```python
from build123d import *

# Parameters (mm, degrees)
SKETCH1_R           = 1.3335
SKETCH1_R_2         = 1.5875
BOSS_EXTRUDE1_DEPTH = 1.651
CHAMFER1_SIZE       = 2.54
SKETCH5_R           = 4.191
CUT_EXTRUDE5_DEPTH  = 23.382376376


with BuildPart() as part:
    # Sketch1 → Boss-Extrude1 (new body)
    with BuildSketch(Plane(origin=(0, 0, 0), x_dir=(1, 0, 0), z_dir=(0, 1, 0))):
        with BuildLine():
            Line((-5.567119422, 8.9535), (5.567119422, 8.9535))
            ThreePointArc((5.567119422, 8.9535), (6.35, 6.5405), (7.132880578, 8.9535))
            Line((7.132880578, 8.9535), (20.447, 8.9535))
            Line((20.447, 8.9535), (20.447, -8.9535))
            Line((20.447, -8.9535), (7.132880578, -8.9535))
            ThreePointArc((7.132880578, -8.9535), (6.35, -6.5405), (5.567119422, -8.9535))
            Line((5.567119422, -8.9535), (-5.567119422, -8.9535))
            ThreePointArc((-5.567119422, -8.9535), (-6.35, -6.5405), (-7.132880578, -8.9535))
            Line((-7.132880578, -8.9535), (-20.447, -8.9535))
            Line((-20.447, -8.9535), (-20.447, 8.9535))
            Line((-20.447, 8.9535), (-7.132880578, 8.9535))
            ThreePointArc((-7.132880578, 8.9535), (-6.35, 6.5405), (-5.567119422, 8.9535))
        make_face()
        with Locations(Location((-17.8308, 5.6769, 0), (0, 0, 90))):
            Circle(SKETCH1_R, mode=Mode.SUBTRACT)
        with Locations(Location((17.8308, 5.6769, 0), (0, 0, 90))):
            Circle(SKETCH1_R, mode=Mode.SUBTRACT)
        with Locations(Location((17.8308, -5.6769, 0), (0, 0, 90))):
            Circle(SKETCH1_R, mode=Mode.SUBTRACT)
        with Locations(Location((-17.8308, -5.6769, 0), (0, 0, 90))):
            Circle(SKETCH1_R, mode=Mode.SUBTRACT)
        with Locations(Location((-10.414, 5.6769, 0), (0, 0, 90))):
            Circle(SKETCH1_R_2, mode=Mode.SUBTRACT)
        with Locations(Location((10.414, 5.6769, 0), (0, 0, 90))):
            Circle(SKETCH1_R_2, mode=Mode.SUBTRACT)
        with Locations(Location((10.414, -5.6769, 0), (0, 0, 90))):
            Circle(SKETCH1_R_2, mode=Mode.SUBTRACT)
        with Locations(Location((-10.414, -5.6769, 0), (0, 0, 90))):
            Circle(SKETCH1_R_2, mode=Mode.SUBTRACT)
    extrude(amount=BOSS_EXTRUDE1_DEPTH)

    # Chamfer1
    chamfer1_edges = [part.edges().sort_by_distance(p)[0] for p in [
        (20.447, 0.8255, -8.9535),
        (20.447, 0.8255, 8.9535),
        (-20.447, 0.8255, 8.9535),
        (-20.447, 0.8255, -8.9535),
    ]]
    chamfer(chamfer1_edges, length=CHAMFER1_SIZE)

    # Sketch5 → Cut-Extrude5 (cut, through all)
    with BuildSketch(Plane(origin=(0, 1.651, 0), x_dir=(1, 0, 0), z_dir=(0, 1, 0))):
        with Locations(Location((-14.0335, 0, 0), (0, 0, 270))):
            Circle(SKETCH5_R)
        with BuildLine():
            Line((6.106574162, -2.159), (11.705551547, -2.159))
            ThreePointArc((11.705551547, -2.159), (17.2085, 0), (11.705551547, 2.159))
            Line((11.705551547, 2.159), (6.106574162, 2.159))
            ThreePointArc((6.106574162, 2.159), (-6.477, 0), (6.106574162, -2.159))
        make_face()
    extrude(amount=-CUT_EXTRUDE5_DEPTH, mode=Mode.SUBTRACT)


solid = part.part
```
Could you check a few things on this model? Use its own coordinates, in mm. A direction names the side the tool comes from. Coordinates: 2 decimals unless noted, no trailing zeros. Write each loop counter-clockwise with the first axis right and the second up, starting at its lowest first coordinate (ties: lowest second). Pieces come first, ordered by that corner, then holes. Notation, with made-up numbers: (19.5, -38.75) -> (24.5, -38.75) arc R28 cw to (24.5, -1.75) -> close; hole circle Ø11 at (-19, 59). An arc over 180 degrees is marked (long way). Return JSON: item names as keys, results as strings.
(1) I need wall thicknesses on L1, parallel to Z at x = 10.5, y = 0.85; L2, parallel to X at y = 0.25, z = 0; L3, parallel to X at y = 1, z = -5.5. Which ranges of each line are inside material? Lowest first, please.
Numbers:
{"L1": "z = -8.95 to -7.26, -4.09 to -2.16, 2.16 to 4.09, 7.26 to 8.95", "L2": "x = -20.45 to -18.22, -9.84 to -6.48, 17.21 to 20.45", "L3": "x = -20.45 to -19.15, -16.51 to -11.99, -8.84 to -3.42, 3.42 to 8.84, 11.99 to 16.51, 19.15 to 20.45"}
(2) Which directions (+Z, -Z, +X, -X, +Y, -Y) give clear straight access to the entire face, cutting with the end or side of a thin tool? Please do faces 4 (the flat face through (9, 1, 2.159)), 5 (the flat face through (13, 1, 8.954)).
Numbers:
{"face 4": "+Y, -Y", "face 5": "+Z, +X, -X, +Y, -Y"}
(3) Imagine slicing it at A-A, the plane x = 0. Please give me the cut outline in (y, z).
Numbers:
{"outline": "(0, -8.95) -> (1.65, -8.95) -> (1.65, -6.48) -> (0, -6.48) -> close; (0, 6.48) -> (1.65, 6.48) -> (1.65, 8.95) -> (0, 8.95) -> close"}
(4) We'd pull the mould along Z, two halves only. Please class faces 1 (the flat face through (12, 1, -8.954)), 2 (the flat face through (-19.16, 0.81, 7.7)), 3 (the flat face through (9, 1, -2.159)): +Z half, -Z half, draft (parallel to the pull), parting line (faces both ways), or undercut.
Numbers:
{"face 1": "-Z half", "face 2": "+Z half", "face 3": "undercut"}
(5) Imagine slicing it at B-B, the plane z = 0. Please give me the cut outline in (x, y), then the cut area to 3 significant figures.
Numbers:
{"outline": "(-20.45, 0) -> (-18.22, 0) -> (-18.22, 1.65) -> (-20.45, 1.65) -> close; (-9.84, 0) -> (-6.48, 0) -> (-6.48, 1.65) -> (-9.84, 1.65) -> close; (17.21, 0) -> (20.45, 0) -> (20.45, 1.65) -> (17.21, 1.65) -> close", "area": "14.6 mm2"}
(6) Imagine slicing it at D-D, the plane y = 0.65. Count the separate pieces of the cut face and the enclosed holes in it, then the cut area to 3 significant figures.
Numbers:
{"separate pieces": "1", "enclosed holes": "10", "area": "405 mm2"}
(7) Imagine slicing it at C-C, the plane z = 5. Please give me the cut outline in (x, y).
Numbers:
{"outline": "(-20.45, 0) -> (-18.98, 0) -> (-18.98, 1.65) -> (-20.45, 1.65) -> close; (-16.68, 0) -> (-11.85, 0) -> (-11.85, 1.65) -> (-16.68, 1.65) -> close; (-8.98, 0) -> (-4.12, 0) -> (-4.12, 1.65) -> (-8.98, 1.65) -> close; (4.12, 0) -> (8.98, 0) -> (8.98, 1.65) -> (4.12, 1.65) -> close; (11.85, 0) -> (16.68, 0) -> (16.68, 1.65) -> (11.85, 1.65) -> close; (18.98, 0) -> (20.45, 0) -> (20.45, 1.65) -> (18.98, 1.65) -> close"}
